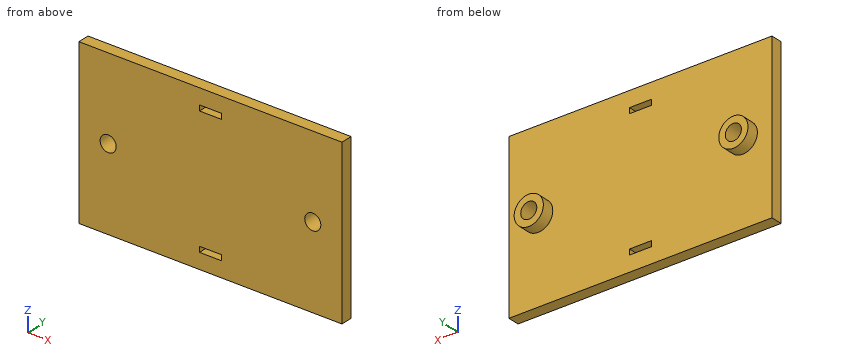
```python
from build123d import *

# Parameters (mm, degrees)
PLATE_START      = 92.57
PLATE_SKETCH_W   = 72
PLATE_SKETCH_H   = 45
PLATE_SKETCH_R   = 2.2
PLATE_SKETCH_W_2 = 6
PLATE_SKETCH_H_2 = 1.5
PLATE_DEPTH      = 3.18
PADS_START       = 95.75
PADS_SKETCH_R    = 4
PADS_SKETCH_R_2  = 2.2
PADS_DEPTH       = 3.3


with BuildPart() as part:
    # Plate Sketch → Plate (new body)
    with BuildSketch(Plane(origin=(0, 0, 0), x_dir=(1, 0, 0), z_dir=(0, 1, 0)).offset(PLATE_START)):
        Rectangle(PLATE_SKETCH_W, PLATE_SKETCH_H)
        with Locations(Location((-28, 0, 0), (0, 0, 270))):
            Circle(PLATE_SKETCH_R, mode=Mode.SUBTRACT)
        with Locations(Location((28, 0, 0), (0, 0, 270))):
            Circle(PLATE_SKETCH_R, mode=Mode.SUBTRACT)
        with Locations((0, 17.5)):
            Rectangle(PLATE_SKETCH_W_2, PLATE_SKETCH_H_2, mode=Mode.SUBTRACT)
        with Locations((0, -17.5)):
            Rectangle(PLATE_SKETCH_W_2, PLATE_SKETCH_H_2, mode=Mode.SUBTRACT)
    extrude(amount=PLATE_DEPTH)

    # Pads Sketch → Pads (add)
    # profile 1 of 2: a face of its own
    with BuildSketch(Plane(origin=(0, 0, 0), x_dir=(1, 0, 0), z_dir=(0, 1, 0)).offset(PADS_START)):
        with Locations(Location((-28, 0, 0), (0, 0, 90))):
            Circle(PADS_SKETCH_R)
        with Locations(Location((-28, 0, 0), (0, 0, 270))):
            Circle(PADS_SKETCH_R_2, mode=Mode.SUBTRACT)
    # profile 2 of 2: a face of its own
    with BuildSketch(Plane(origin=(0, 0, 0), x_dir=(1, 0, 0), z_dir=(0, 1, 0)).offset(PADS_START)):
        with Locations(Location((28, 0, 0), (0, 0, 90))):
            Circle(PADS_SKETCH_R)
        with Locations(Location((28, 0, 0), (0, 0, 270))):
            Circle(PADS_SKETCH_R_2, mode=Mode.SUBTRACT)
    extrude(amount=PADS_DEPTH)


solid = part.part
```
Input: part model. Units: mm. Frame: model coordinates. Round coordinates to 2 decimals unless told otherwise and drop trailing zeros. Loops run counter-clockwise (first coordinate to the right, second up) from the corner with the lowest first, then second, coordinate; pieces in that order, holes last. Notation, with made-up numbers: M 61,-18 L 120,-18 A32 cw 120,9 Z; hole C -15.75,16 d6. An arc over 180 degrees is marked long. Answer in a Markdown table with one row per item. Add a question column.
1. Section D-D (x = 9). Output: boundary loops of the cut face in (y, z), and give its area (3 significant figures).
2. Section B-B (z = 0). Output: boundary loops of the cut face in (x, y).
3. Section A-A (x = -28). Output: boundary loops of the cut face in (y, z).
4. Section C-C (z = 12). Output: boundary loops of the cut face in (x, y).
5. Ray query, probe 1 along Z at (x, y) = (2, 93.5); probe 2 along X at (y, z) = (95.5, 0); probe 3 along X at (y, z) = (96, 0). Return the intervals inside material, ascending.
6. Contact query for flat-ended pins moving along their axis: pin 1 (3 mm diameter, centred on x = 5.5, z = 0, fed in from +Y); pin 2 (5 mm diameter, centred on x = 28, z = 0, fed in from +Y). Output: stop coordinate, or through.
Values follow:
| question | item | result |
|---|---|---|
| 1 | outline | M 92.57,-22.5 L 95.75,-22.5 L 95.75,22.5 L 92.57,22.5 Z |
| 1 | area | 143 mm^2 |
| 2 | outline | M -36,92.57 L -30.2,92.57 L -30.2,99.05 L -32,99.05 L -32,95.75 L -36,95.75 Z; M -25.8,92.57 L 25.8,92.57 L 25.8,99.05 L 24,99.05 L 24,95.75 L -24,95.75 L -24,99.05 L -25.8,99.05 Z; M 30.2,92.57 L 36,92.57 L 36,95.75 L 32,95.75 L 32,99.05 L 30.2,99.05 Z |
| 3 | outline | M 92.57,-22.5 L 95.75,-22.5 L 95.75,-4 L 99.05,-4 L 99.05,-2.2 L 92.57,-2.2 Z; M 92.57,2.2 L 99.05,2.2 L 99.05,4 L 95.75,4 L 95.75,22.5 L 92.57,22.5 Z |
| 4 | outline | M -36,92.57 L 36,92.57 L 36,95.75 L -36,95.75 Z |
| 5 | probe 1 | -22.5 to -18.25, -16.75 to 16.75, 18.25 to 22.5 |
| 5 | probe 2 | -36 to -30.2, -25.8 to 25.8, 30.2 to 36 |
| 5 | probe 3 | -32 to -30.2, -25.8 to -24, 24 to 25.8, 30.2 to 32 |
| 6 | pin 1 | y = 95.75 |
| 6 | pin 2 | y = 99.05 |
